Verification items for the finished model (mm, model axes). Coordinates: 2 decimals unless noted, no trailing zeros. Order: outer loops, then holes, each group sorted by start corner. A loop starts at its lowest first (then second) coordinate and runs counter-clockwise, first axis right, second up. Notation, with made-up numbers: (17, 58.25) - (41, 58.25) arc R25 cw to (41, 97.25) - close; hole circle Ø5 at (78, -31). An arc over 180 degrees is marked (long way). Answer as CSV lines item,"result". Start each with the question number.
1. Section check B-B (y = -1). Record the cut outline in (x, z), and give its area (3 significant figures).
2. Go/stop test with flat-tipped pins: pin 1 (3 mm diameter, centred on x = 15, y = 2.5, fed in from -Z); pin 2 (2 mm diameter, centred on x = 28.58, y = 9.13, fed in from +Z). Record where each tip stops, or that it passes through.
3. Section check A-A (x = 0). Record the cut outline in (y, z).
4. Material ranges on L1, parallel to Y at x = 0, z = 0.25; L2, parallel to X at y = 9.75, z = 0.5; L3, parallel to X at y = 1.5, z = 0.2, recorded low to high. Write a range as [from, to].
5. Section check D-D (z = 0.45). Record the cut outline in (x, y) (1 decimal), and give its area (3 significant figures).
6. Section check C-C (y = 6.75). Record the cut outline in (x, z), and give its area (3 significant figures).
from build123d import *

# Parameters (mm, degrees)
SKETCH1_R           = 1.7859375
BOSS_EXTRUDE1_DEPTH = 0.8128


with BuildPart() as part:
    # Sketch1 → Boss-Extrude1 (new body)
    with BuildSketch(Plane.XY):
        with BuildLine():
            ThreePointArc((5.113201981, -2.174184805), (6.429738102, -0.592725316), (8.400260413, 0))
            Line((8.400260413, 0), (20.174739587, 0))
            ThreePointArc((20.174739587, 0), (22.145261898, -0.592725316), (23.461798019, -2.174184805))
            ThreePointArc((23.461798019, -2.174184805), (31.640256951, -4.634232826), (32.576636291, 3.854714135))
            ThreePointArc((32.576636291, 3.854714135), (31.636446649, 5.685103372), (31.862058429, 7.730434799))
            ThreePointArc((31.862058429, 7.730434799), (29.288207259, 12.628071631), (25.003125, 9.128125))
            ThreePointArc((25.003125, 9.128125), (23.956947034, 6.602427966), (21.43125, 5.55625))
            Line((21.43125, 5.55625), (7.14375, 5.55625))
            ThreePointArc((7.14375, 5.55625), (4.618052966, 6.602427966), (3.571875, 9.128125))
            ThreePointArc((3.571875, 9.128125), (-0.713207259, 12.628071631), (-3.287058429, 7.730434799))
            ThreePointArc((-3.287058429, 7.730434799), (-3.061446655, 5.68510334), (-4.001636336, 3.854714088))
            ThreePointArc((-4.001636336, 3.854714088), (-3.065256924, -4.634232844), (5.113201981, -2.174184805))
        make_face()
        Circle(SKETCH1_R, mode=Mode.SUBTRACT)
        with Locations((28.575, 0)):
            Circle(SKETCH1_R, mode=Mode.SUBTRACT)
        with Locations((0, 9.128125)):
            Circle(SKETCH1_R, mode=Mode.SUBTRACT)
        with Locations((28.575, 9.128125)):
            Circle(SKETCH1_R, mode=Mode.SUBTRACT)
    extrude(amount=BOSS_EXTRUDE1_DEPTH)


solid = part.part
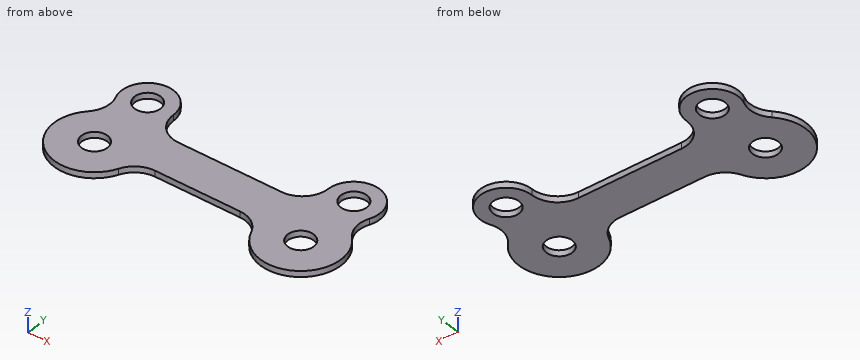
Evaluation:
1,outline,"(-5.47, 0) - (-1.48, 0) - (-1.48, 0.81) - (-5.47, 0.81) - close; (1.48, 0) - (5.92, 0) - (5.92, 0.81) - (1.48, 0.81) - close; (22.65, 0) - (27.1, 0) - (27.1, 0.81) - (22.65, 0.81) - close; (30.05, 0) - (34.04, 0) - (34.04, 0.81) - (30.05, 0.81) - close"
1,area,"13.7 mm²"
2,pin 1,"stops at z = 0"
2,pin 2,"passes through"
3,outline,"(-5.56, 0) - (-1.79, 0) - (-1.79, 0.81) - (-5.56, 0.81) - close; (1.79, 0) - (7.34, 0) - (7.34, 0.81) - (1.79, 0.81) - close; (10.91, 0) - (12.7, 0) - (12.7, 0.81) - (10.91, 0.81) - close"
4,L1,"y = [-5.56, -1.79], [1.79, 7.34], [10.91, 12.7]"
4,L2,"x = [-3.52, -1.67], [1.67, 3.52], [25.06, 26.9], [30.25, 32.09]"
4,L3,"x = [-5.35, -0.97], [0.97, 27.61], [29.54, 33.92]"
5,outline,"(-4, 3.9) arc R5.6 ccw (long way) to (5.1, -2.2) arc R3.6 cw to (8.4, 0) - (20.2, 0) arc R3.6 cw to (23.5, -2.2) arc R5.6 ccw (long way) to (32.6, 3.9) arc R3.6 cw to (31.9, 7.7) arc R3.6 ccw (long way) to (25, 9.1) arc R3.6 cw to (21.4, 5.6) - (7.1, 5.6) arc R3.6 cw to (3.6, 9.1) arc R3.6 ccw (long way) to (-3.3, 7.7) arc R3.6 cw to start; hole circle Ø3.6 at (0, 0); hole circle Ø3.6 at (0, 9.1); hole circle Ø3.6 at (28.6, 0); hole circle Ø3.6 at (28.6, 9.1)"
5,area,"363 mm²"
6,outline,"(-3.03, 0) - (4.48, 0) - (4.48, 0.81) - (-3.03, 0.81) - close; (24.1, 0) - (31.6, 0) - (31.6, 0.81) - (24.1, 0.81) - close"
6,area,"12.2 mm²"
